For this review, take the finished solid that the model builds, in its own axes (mm). A direction names the side the tool comes from. Round coordinates to 2 decimals unless told otherwise and drop trailing zeros. Write each loop counter-clockwise with the first axis right and the second up, starting at its lowest first coordinate (ties: lowest second). Pieces come first, ordered by that corner, then holes. Notation, with made-up numbers: (83.25, 72.5) -> (120.25, 72.5) arc R25 cw to (120.25, 94.5) -> close; hole circle Ø8 at (-38, 48.5). An arc over 180 degrees is marked (long way). Answer in a Markdown table with one row per item.
from build123d import *

# Parameters (mm, degrees)
F0_R          = 4.5
F1_DEPTH      = 4
F1_DEPTH_BACK = 15
F0_W          = 13
F0_H          = 15
F2_DEPTH      = 15
F3_D          = 2.2
F3_DEPTH      = 8
F3_TIP        = 0.6609466809
F4_D          = 8.5
F4_DEPTH      = 8
F4_TIP        = 2.5536576309
F6_D          = 2.5
F6_DEPTH      = 5
F6_TIP        = 0.7510757738


with BuildPart() as f1:
    # F0 (on Front) → F1 (new body, two sides)
    with BuildSketch(Plane.XZ) as f1_sk:
        with Locations((0, 0.5)):
            Circle(F0_R)
    extrude(amount=F1_DEPTH)
    extrude(f1_sk.sketch, amount=-F1_DEPTH_BACK)

    # F0 (on Front) → F2 (join)
    with BuildSketch(Plane.XZ):
        Rectangle(F0_W, F0_H)
        with Locations((0, 0.5)):
            Circle(F0_R, mode=Mode.SUBTRACT)
    extrude(amount=-F2_DEPTH)

    # F3
    with Locations(Plane.XZ):
        with Locations((4.5, 5), (4.5, -4), (-4.5, 5), (-4.5, -4)):
            Hole(F3_D / 2, depth=F3_DEPTH)
            with Locations((0, 0, -(F3_DEPTH + F3_TIP / 2))):  # 118° drill point
                Cone(0, F3_D / 2, F3_TIP, mode=Mode.SUBTRACT)

    # F4 (one way)
    with BuildSketch(Plane(origin=(0, 0, 0), x_dir=(1, 0, 0), z_dir=(0, 1, 0))):
        with Locations((0, -0.5)):
            Circle(F4_D / 2)
    extrude(amount=-F4_DEPTH, mode=Mode.SUBTRACT)
    with Locations(Plane(origin=(0, 0, 0), x_dir=(1, 0, 0), z_dir=(0, 1, 0))):
        with Locations((0, -0.5)):
            with Locations((0, 0, -(F4_DEPTH + F4_TIP / 2))):  # 118° drill point
                Cone(0, F4_D / 2, F4_TIP, mode=Mode.SUBTRACT)

    # F6
    with Locations(Plane(origin=(0, 0, -7.5), x_dir=(1, 0, 0), z_dir=(0, 0, -1))):
        with Locations((-3.25, -6), (3.25, -6)):
            Hole(F6_D / 2, depth=F6_DEPTH)
            with Locations((0, 0, -(F6_DEPTH + F6_TIP / 2))):  # 118° drill point
                Cone(0, F6_D / 2, F6_TIP, mode=Mode.SUBTRACT)


solid = f1.part
1) Mouldability with a two-part tool opening along X and no side actions: class faces 4 (the cylindrical face through (-0.59, -2.03, 4.96)), 5 (the flat face through (6.5, 7, 0)), 6 (the conical face through (-3.5, 6, -1.9)) as pulls with the +X half, pulls with the -X half, needs draft (parallel to the pull), parting line crosses it, or undercut.
Solved:
| item | result |
|---|---|
| face 4 | parting line crosses it |
| face 5 | pulls with the +X half |
| face 6 | undercut |
2) Consider section A-A on z = -6. State the section outline as (x, y) points, then the cut area to 3 significant figures.
Solved:
| item | result |
|---|---|
| outline | (-6.5, 0) -> (6.5, 0) -> (6.5, 15) -> (-6.5, 15) -> close; hole circle Ø2.5 at (-3.25, 6); hole circle Ø2.5 at (3.25, 6) |
| area | 185 mm² |
3) For line 1 (X direction, y = 4.5, z = 5); line 2 (Z direction, x = 4.5, y = 6.5); line 3 (Y direction, x = 3.25, z = -3.9), list the stretches that pass through material, from the lowest coordinate up. Write a range as [from, to].
Solved:
| item | result |
|---|---|
| line 1 | [-6.5, -5.6], [-3.4, 3.4], [5.6, 6.5] |
| line 2 | [-7.5, -5.1], [-2.9, 3.9], [6.1, 7.5] |
| line 3 | [0, 4.75], [7.25, 15] |
4) Consider section C-C on z = 1.5. State the section outline as (x, y) points.
Solved:
| item | result |
|---|---|
| outline | (-6.5, 0) -> (-4.39, 0) -> (-4.39, -4) -> (-4.13, -4) -> (-4.13, 0) -> (4.13, 0) -> (4.13, -4) -> (4.39, -4) -> (4.39, 0) -> (6.5, 0) -> (6.5, 15) -> (-6.5, 15) -> close |
5) Consider section D-D on z = -2. State the section outline as (x, y) points.
Solved:
| item | result |
|---|---|
| outline | (-6.5, 0) -> (-3.74, 0) -> (-3.74, -4) -> (-3.44, -4) -> (-3.44, 0) -> (3.44, 0) -> (3.44, -4) -> (3.74, -4) -> (3.74, 0) -> (6.5, 0) -> (6.5, 15) -> (-6.5, 15) -> close; hole circle Ø0.84 at (-3.25, 6); hole circle Ø0.84 at (3.25, 6) |
6) Clearance check with flat-ended pins moving along their axes: pin 1 Ø2 at (x, z) = (-4.5, -4) entering from -Y; pin 2 Ø2 at (x, y) = (-3.25, 6) entering from -Z; pin 3 Ø3 at (x, z) = (-4.5, 5) entering from -Y. State where each tip first meets the part, or that it passes through.
Solved:
| item | result |
|---|---|
| pin 1 | y = 8.06 |
| pin 2 | z = -2.35 |
| pin 3 | y = 0 |
7) For faces 1 (the cylindrical face through (2, 6, -5)), 2 (the flat face through (-6.5, 7, 0)), 3 (the cylindrical face through (-0.553, -1.972, -3.714)), list the 3-axis set-ups (+Z, -Z, +X, -X, +Y, -Y) from which the entire face can be reached by the end or side of a thin tool; tool diameter is ignored.
Solved:
| item | result |
|---|---|
| face 1 | -Z |
| face 2 | +Z, -Z, -X, +Y, -Y |
| face 3 | -Y |
8) Consider section B-B on x = 0. State the section outline as (y, z) points.
Solved:
| item | result |
|---|---|
| outline | (-4, -4) -> (0, -4) -> (0, -7.5) -> (15, -7.5) -> (15, 7.5) -> (0, 7.5) -> (0, 5) -> (-4, 5) -> (-4, 4.75) -> (0, 4.75) -> (0, -3.75) -> (-4, -3.75) -> close |
